Check sheet for the modelled part. Datum: model origin and axes. Units: mm. A direction names the side the tool comes from. Give positions to 0.01 mm unless a question says otherwise; leave off trailing zeros. Order: outer loops, then holes, each group sorted by start corner. A loop starts at its lowest first (then second) coordinate and runs counter-clockwise, first axis right, second up. Notation, with made-up numbers: (-4, 25) - (32, 25) arc R21 cw to (32, 53) - close; hole circle Ø4 at (4, -34.75). An arc over 180 degrees is marked (long way). Answer in a Markdown table with one row per item.
from build123d import *

# Parameters (mm, degrees)
BOSS_EXTRUDE5_OUTLINE_W   = 80
BOSS_EXTRUDE5_OUTLINE_H   = 162
BOSS_EXTRUDE5_OUTLINE_W_2 = 1.57
BOSS_EXTRUDE5_OUTLINE_H_2 = 27
BOSS_EXTRUDE5_DEPTH       = 3
SKETCH8_R                 = 2.2
SKETCH8_R_2               = 2.02
CUT_EXTRUDE1_DEPTH        = 10
CUT_EXTRUDE2_DEPTH        = 10
CUT_EXTRUDE2_DEPTH_BACK   = 3
SKETCH9_W                 = 3
SKETCH9_H                 = 6
SKETCH9_W_2               = 6
SKETCH9_H_2               = 3
SKETCH9_W_3               = 1.02
SKETCH9_H_3               = 8.89
SKETCH9_W_4               = 8.89
SKETCH9_H_4               = 1.02
SKETCH9_W_5               = 4.655263111
SKETCH9_H_5               = 28.36
FILLET3_R                 = 4


# Read off the part's stored shape, not the designer's step: Boss-Extrude5
with BuildPart() as part:
    # Boss-Extrude5 outline → Boss-Extrude5 (new body)
    with BuildSketch(Plane(origin=(0, 0, 0), x_dir=(1, 0, 0), z_dir=(0, 1, 0))):
        with Locations((-31.485263111, -108.03530565)):
            Rectangle(BOSS_EXTRUDE5_OUTLINE_W, BOSS_EXTRUDE5_OUTLINE_H)
        with BuildLine():
            Line((-34.801887901, -89.53530565), (-28.16863832, -89.53530565))
            ThreePointArc((-28.16863832, -89.53530565), (-25.485263111, -94.53530565), (-28.16863832, -99.53530565))
            Line((-28.16863832, -99.53530565), (-34.801887901, -99.53530565))
            ThreePointArc((-34.801887901, -99.53530565), (-37.485263111, -94.53530565), (-34.801887901, -89.53530565))
        make_face(mode=Mode.SUBTRACT)
        with BuildLine():
            Line((-30.985263111, -86.621331054), (-30.985263111, -87.75530565))
            Line((-30.985263111, -87.75530565), (-31.985263111, -87.75530565))
            Line((-31.985263111, -87.75530565), (-31.985263111, -86.621331054))
            ThreePointArc((-31.985263111, -86.621331054), (-31.485263111, -84.75530565), (-30.985263111, -86.621331054))
        make_face(mode=Mode.SUBTRACT)
        with BuildLine():
            Line((-25.885263111, -82.98030565), (-37.085263111, -82.98030565))
            ThreePointArc((-37.085263111, -82.98030565), (-37.438816501, -82.833859041), (-37.585263111, -82.48030565))
            Line((-37.585263111, -82.48030565), (-37.585263111, -60.78030565))
            ThreePointArc((-37.585263111, -60.78030565), (-37.438816502, -60.42675226), (-37.085263111, -60.28030565))
            Line((-37.085263111, -60.28030565), (-25.885263111, -60.28030565))
            ThreePointArc((-25.885263111, -60.28030565), (-25.53170972, -60.426752259), (-25.385263111, -60.78030565))
            Line((-25.385263111, -60.78030565), (-25.385263111, -82.48030565))
            ThreePointArc((-25.385263111, -82.48030565), (-25.53170972, -82.833859041), (-25.885263111, -82.98030565))
        make_face(mode=Mode.SUBTRACT)
        with Locations((-13.090263111, -82.857662255)):
            Rectangle(BOSS_EXTRUDE5_OUTLINE_W_2, BOSS_EXTRUDE5_OUTLINE_H_2, mode=Mode.SUBTRACT)
        with BuildLine():
            ThreePointArc((-30.985263111, -56.639280246), (-31.485263111, -58.50530565), (-31.985263111, -56.639280246))
            Line((-31.985263111, -56.639280246), (-31.985263111, -55.50530565))
            Line((-31.985263111, -55.50530565), (-30.985263111, -55.50530565))
            Line((-30.985263111, -55.50530565), (-30.985263111, -56.639280246))
        make_face(mode=Mode.SUBTRACT)
    extrude(amount=BOSS_EXTRUDE5_DEPTH)

    # Sketch8 → Cut-Extrude1 (cut)
    with BuildSketch(Plane(origin=(0, 3, 0), x_dir=(1, 0, 0), z_dir=(0, 1, 0))):
        with Locations(Location((-43.415263111, -118.95530565, 0), (0, 0, 270))):
            Circle(SKETCH8_R)
        with Locations(Location((-19.555263111, -118.95530565, 0), (0, 0, 270))):
            Circle(SKETCH8_R)
        with Locations(Location((-19.555263111, -158.99530565, 0), (0, 0, 270))):
            Circle(SKETCH8_R_2)
        with Locations(Location((-43.415263111, -158.99530565, 0), (0, 0, 270))):
            Circle(SKETCH8_R)
    extrude(amount=-CUT_EXTRUDE1_DEPTH, mode=Mode.SUBTRACT)

    # Sketch9 → Cut-Extrude2 (cut, two sides: drawn at the far end of the back side and taken through both)
    with BuildSketch(Plane(origin=(0, 3, 0), x_dir=(1, 0, 0), z_dir=(0, 1, 0)).offset(-CUT_EXTRUDE2_DEPTH_BACK)):
        with Locations((-52.985263111, -183.53530565)):
            Rectangle(SKETCH9_W, SKETCH9_H)
        with Locations((-9.985263111, -183.53530565)):
            Rectangle(SKETCH9_W, SKETCH9_H)
        with Locations((-9.985263111, -138.53530565)):
            Rectangle(SKETCH9_W, SKETCH9_H)
        with Locations((-52.985263111, -138.53530565)):
            Rectangle(SKETCH9_W, SKETCH9_H)
        Polygon((-37.585263111, -81.53530565), (-40.585263111, -81.53530565), (-40.585263111, -87.53530565), (-37.585263111, -87.53530565), (-37.585263111, -82.48030565), align=None)
        Polygon((-25.385263111, -87.53530565), (-22.385263111, -87.53530565), (-22.385263111, -81.53530565), (-25.385263111, -81.53530565), (-25.385263111, -82.48030565), align=None)
        with Locations((-44.485263111, -185.03530565)):
            Rectangle(SKETCH9_W_2, SKETCH9_H_2)
        with Locations((-18.485263111, -185.03530565)):
            Rectangle(SKETCH9_W_2, SKETCH9_H_2)
        with Locations((-44.485263111, -137.03530565)):
            Rectangle(SKETCH9_W_2, SKETCH9_H_2)
        with Locations((-18.485263111, -137.03530565)):
            Rectangle(SKETCH9_W_2, SKETCH9_H_2)
        with Locations((-69.465263111, -71.94030565)):
            Rectangle(SKETCH9_W_3, SKETCH9_H_3)
        with Locations((-31.485263111, -29.05530565)):
            Rectangle(SKETCH9_W_4, SKETCH9_H_4)
        with Locations((6.494736889, -71.94030565)):
            Rectangle(SKETCH9_W_3, SKETCH9_H_3)
        with Locations((-64.240263111, -186.51530565)):
            Rectangle(SKETCH9_W_4, SKETCH9_H_4)
        with Locations((1.269736889, -186.51530565)):
            Rectangle(SKETCH9_W_4, SKETCH9_H_4)
        Polygon((0, -97.31530565), (-4.655263111, -97.31530565), (-4.655263111, -144.03530565), (7.584736889, -144.03530565), (7.584736889, -97.31530565), align=None)
        with Locations((-2.327631556, -83.13530565)):
            Rectangle(SKETCH9_W_5, SKETCH9_H_5)
        with Locations((-43.025263111, -37.07530565)):
            Rectangle(SKETCH9_W_2, SKETCH9_H_2)
        with Locations((-19.945263111, -37.07530565)):
            Rectangle(SKETCH9_W_2, SKETCH9_H_2)
        Polygon((-16.945263111, -27.03530565), (8.514736889, -64.49530565), (8.514736889, -27.03530565), align=None)
        Polygon((-71.485263111, -27.03530565), (-71.485263111, -64.49530565), (-46.025263111, -27.03530565), align=None)
    extrude(amount=CUT_EXTRUDE2_DEPTH + CUT_EXTRUDE2_DEPTH_BACK, mode=Mode.SUBTRACT)

    # Fillet3
    fillet3_edges = [part.edges().sort_by_distance(p)[0] for p in [
        (-16.945263111, 1.5, 27.03530565),
        (8.514736889, 1.5, 64.49530565),
        (-71.485263111, 1.5, 64.49530565),
        (-46.025263111, 1.5, 27.03530565),
        (-71.485263111, 1.5, 189.03530565),
        (8.514736889, 1.5, 189.03530565),
    ]]
    fillet(fillet3_edges, radius=FILLET3_R)


solid = part.part
(1) Gauge pin test, flat ends, axial feed: P1, Ø0.8, axis at y = 2, z = 186.5, coming from the -X side; P2, Ø0.5, axis at x = 6.5, y = 1.5, coming from the -Z side; P3, Ø1.2, axis at y = 1, z = 56, coming from the +X side; P4, Ø4, axis at x = -43.42, z = 159, coming from the -Y side. Record the tip position at first contact, or that the pin passes through.
Geometry says:
| item | result |
|---|---|
| P1 | x = -71.34 |
| P2 | z = 61.16 |
| P3 | x = 3.15 |
| P4 | through |
(2) Access from +Z, -Z, +X, -X, +Y, -Y to the whole of each face (thin tool, end or side, straight path). Record for faces 1 (the flat face through (-53, 1, 141.535)), 2 (the cylindrical face through (7.312, 1.521, 187.895)).
Geometry says:
| item | result |
|---|---|
| face 1 | +Y, -Y |
| face 2 | +Z, +X, +Y, -Y |
(3) Cross-section at A-A, the plane z = 137. Record the cut outline in (x, y).
Geometry says:
| item | result |
|---|---|
| outline | (-71.49, 0) - (-54.49, 0) - (-54.49, 3) - (-71.49, 3) - close; (-51.49, 0) - (-47.49, 0) - (-47.49, 3) - (-51.49, 3) - close; (-41.49, 0) - (-21.49, 0) - (-21.49, 3) - (-41.49, 3) - close; (-15.49, 0) - (-11.49, 0) - (-11.49, 3) - (-15.49, 3) - close; (-8.49, 0) - (-4.66, 0) - (-4.66, 3) - (-8.49, 3) - close; (7.58, 0) - (8.51, 0) - (8.51, 3) - (7.58, 3) - close |
(4) Mould release check, pull along Z, two halves, no side actions. Record for faces 3 (the cylindrical face through (-70.345, 1.521, 187.832)), 4 (the flat face through (-24, 1, 87.535)), 5 (the flat face through (-32, 1, 27.035)): pulls with the +Z half, pulls with the -Z half, needs draft (parallel to the pull), parting line crosses it, or undercut.
Geometry says:
| item | result |
|---|---|
| face 3 | pulls with the +Z half |
| face 4 | undercut |
| face 5 | pulls with the -Z half |
(5) Cross-section at C-C, the plane y = 2.15. Give the number of separate pieces and of enclosed holes in the cut face, then the cut area to 3 significant figures.
Geometry says:
| item | result |
|---|---|
| separate pieces | 1 |
| enclosed holes | 25 |
| area | 10,500 mm² |
(6) Cross-section at B-B, the plane z = 92.5. Record the cut outline in (x, y).
Geometry says:
| item | result |
|---|---|
| outline | (-71.49, 0) - (-37.13, 0) - (-37.13, 3) - (-71.49, 3) - close; (-25.84, 0) - (-13.88, 0) - (-13.88, 3) - (-25.84, 3) - close; (-12.31, 0) - (-4.66, 0) - (-4.66, 3) - (-12.31, 3) - close; (0, 0) - (8.51, 0) - (8.51, 3) - (0, 3) - close |
(7) Thickness scan on L1, parallel to X at y = 1.2, z = 88.5; L2, parallel to X at y = 2.1, z = 78.5; L3, parallel to X at y = 1.3, z = 127. Record the ranges inside material, lowest first.
Geometry says:
| item | result |
|---|---|
| L1 | -71.49 to -13.88, -12.31 to -4.66, 0 to 8.51 |
| L2 | -71.49 to -37.59, -25.39 to -13.88, -12.31 to -4.66, 0 to 8.51 |
| L3 | -71.49 to -4.66, 7.58 to 8.51 |
